```python
from build123d import *

# Parameters (mm, degrees)
BOSS_EXTRUDE1_DEPTH = 510
SKETCH2_R           = 2.75
CUT_EXTRUDE1_DEPTH  = 5


with BuildPart() as part:
    # Sketch1 → Boss-Extrude1 (new body)
    with BuildSketch(Plane.XY):
        Polygon((0, 0), (-50, 0), (-50, 2), (-2, 2), (-2, 50), (0, 50), align=None)
    extrude(amount=BOSS_EXTRUDE1_DEPTH)

    # Sketch2 → Cut-Extrude1 (cut, symmetric)
    with BuildSketch(Plane(origin=(0, 0, 0), x_dir=(0, 0, -1), z_dir=(1, 0, 0))):
        with Locations((-21.25, 39)):
            Circle(SKETCH2_R)
        with Locations((-63.75, 39)):
            Circle(SKETCH2_R)
        with Locations((-106.25, 39)):
            Circle(SKETCH2_R)
        with Locations((-148.75, 39)):
            Circle(SKETCH2_R)
        with Locations((-191.25, 39)):
            Circle(SKETCH2_R)
        with Locations((-233.75, 39)):
            Circle(SKETCH2_R)
        with Locations((-276.25, 39)):
            Circle(SKETCH2_R)
        with Locations((-318.75, 39)):
            Circle(SKETCH2_R)
        with Locations((-352.5, 39)):
            Circle(SKETCH2_R)
        with Locations((-377.5, 39)):
            Circle(SKETCH2_R)
        with Locations((-402.5, 39)):
            Circle(SKETCH2_R)
        with Locations((-427.5, 39)):
            Circle(SKETCH2_R)
        with Locations((-452.5, 39)):
            Circle(SKETCH2_R)
        with Locations((-477.5, 39)):
            Circle(SKETCH2_R)
        with Locations((-497.5, 39)):
            Circle(SKETCH2_R)
    extrude(amount=CUT_EXTRUDE1_DEPTH, both=True, mode=Mode.SUBTRACT)


solid = part.part
```
For this review, take the finished solid that the model builds, in its own axes (mm). A direction names the side the tool comes from. Round coordinates to 2 decimals unless told otherwise and drop trailing zeros. Write each loop counter-clockwise with the first axis right and the second up, starting at its lowest first coordinate (ties: lowest second). Pieces come first, ordered by that corner, then holes. Notation, with made-up numbers: (-16, -38) - (43, -38) arc R28 cw to (43, -16) - close; hole circle Ø2 at (29.25, 68.5). An arc over 180 degrees is marked (long way). Answer as CSV lines item,"result". Start each with the question number.
(1) For line 1 (Y direction, x = -1.3, z = 21.25); line 2 (Y direction, x = -44, z = 206); line 3 (X direction, y = 33.5, z = 105.5), list the stretches that pass through material, from the lowest coordinate up.
(2) Add section A-A, the plane z = 267.5. State the section outline as (x, y) points.
(3) For pin 1 (7 mm diameter, centred on y = 39, z = 477.5, fed in from -X); pin 2 (10 mm diameter, centred on x = -33.5, z = 86.5, fed in from +Y); pin 3 (4.5 mm diameter, centred on y = 39, z = 427.5, fed in from -X) (1 decimal), all flat-tipped, find the tip position at first contact; note any pin that passes through.
(4) Add section C-C, the plane y = 13. State the section outline as (x, z) points.
(5) Machinability: for faces 1 (the flat face through (-14, 1, 0)), 2 (the flat face through (-2, 26, 251)), which of the approach directions +Z, -Z, +X, -X, +Y, -Y give a long, thin tool a straight path to every point of the face, cutting with its end or side? Answer none if there is none.
(6) Add section B-B, the plane x = -10. State the section outline as (y, z) points, plus the area to 3 significant figures.
From the geometry:
1,line 1,"y = 0 to 36.25, 41.75 to 50"
1,line 2,"y = 0 to 2"
1,line 3,"x = -2 to 0"
2,outline,"(-50, 0) - (0, 0) - (0, 50) - (-2, 50) - (-2, 2) - (-50, 2) - close"
3,pin 1,"stops at x = -2"
3,pin 2,"stops at y = 2"
3,pin 3,"passes through"
4,outline,"(-2, 0) - (0, 0) - (0, 510) - (-2, 510) - close"
5,face 1,"-Z, +X, -X, +Y, -Y"
5,face 2,"+Z, -Z, -X, +Y"
6,outline,"(0, 0) - (2, 0) - (2, 510) - (0, 510) - close"
6,area,"1,020 mm²"
